from build123d import *

# Parameters (mm, degrees)
F1_DEPTH  = 250
F2_R      = 5
F3_DEPTH  = 25
F5_DEPTH  = 25
F7_DEPTH  = 25
F10_DEPTH = 100


with BuildPart() as f1:
    # F0 (on Front) → F1 (new body)
    with BuildSketch(Plane.XZ):
        Polygon((-47.1529836208, 41.1845914816), (-77.1529836208, 41.1845914816), (-77.1529836208, 38.1845914816), (-47.1529836208, 38.1845914816), (-47.1529836208, 11.1845914816), (27.0837845569, -25.3437928188), (45.465561148, -49.0526580248), (47.8364476686, -50.2144803657), (67.8364476686, -50.2144803657), (67.8364476686, -47.2144803657), (47.8364476686, -47.2144803657), (28.3516393422, -22.6248694577), (-44.1529836208, 11.1845914816), (-44.1529836208, 41.1845914816), align=None)
    extrude(amount=F1_DEPTH)

    # F2 (on face) → F3 (cut)
    with BuildSketch(Plane.XY.offset(41.1845914816)):
        with Locations((-61.1529836208, -30)):
            Circle(F2_R)
        with Locations((-61.1529836208, -125)):
            Circle(F2_R)
        with Locations((-61.1529836208, -220)):
            Circle(F2_R)
    extrude(amount=-F3_DEPTH, mode=Mode.SUBTRACT)

    # F4 (on face) → F5 (cut)
    with BuildSketch(Plane.XY.offset(41.1845914816)):
        with BuildLine():
            ThreePointArc((-77.1529836208, -25), (-69.8306531504, -7.3223304703), (-52.1529836208, 0))
            Line((-52.1529836208, 0), (-77.1529836208, 0))
            Line((-77.1529836208, 0), (-77.1529836208, -25))
        make_face()
        with BuildLine():
            Line((-77.1529836208, -250), (-52.1529836208, -250))
            ThreePointArc((-52.1529836208, -250), (-69.8306531504, -242.6776695297), (-77.1529836208, -225))
            Line((-77.1529836208, -225), (-77.1529836208, -250))
        make_face()
    extrude(amount=-F5_DEPTH, mode=Mode.SUBTRACT)

    # F6 (on face) → F7 (cut)
    with BuildSketch(Plane.XY.offset(41.1845914816)):
        with BuildLine():
            Line((-58.6529836208, -40), (-63.6529836208, -40))
            ThreePointArc((-63.6529836208, -40), (-67.1885175267, -41.4644660941), (-68.6529836208, -45))
            Line((-68.6529836208, -45), (-68.6529836208, -110))
            ThreePointArc((-68.6529836208, -110), (-67.1885175267, -113.5355339059), (-63.6529836208, -115))
            Line((-63.6529836208, -115), (-58.6529836208, -115))
            ThreePointArc((-58.6529836208, -115), (-55.1174497148, -113.5355339059), (-53.6529836208, -110))
            Line((-53.6529836208, -110), (-53.6529836208, -45))
            ThreePointArc((-53.6529836208, -45), (-55.1174497148, -41.4644660941), (-58.6529836208, -40))
        make_face()
        with BuildLine():
            Line((-58.6529836208, -135), (-63.6529836208, -135))
            ThreePointArc((-63.6529836208, -135), (-67.1885175267, -136.4644660941), (-68.6529836208, -140))
            Line((-68.6529836208, -140), (-68.6529836208, -205))
            ThreePointArc((-68.6529836208, -205), (-67.1885175267, -208.5355339059), (-63.6529836208, -210))
            Line((-63.6529836208, -210), (-58.6529836208, -210))
            ThreePointArc((-58.6529836208, -210), (-55.1174497148, -208.5355339059), (-53.6529836208, -205))
            Line((-53.6529836208, -205), (-53.6529836208, -140))
            ThreePointArc((-53.6529836208, -140), (-55.1174497148, -136.4644660941), (-58.6529836208, -135))
        make_face()
    extrude(amount=-F7_DEPTH, mode=Mode.SUBTRACT)

    # F9 (on offset) → F10 (cut)
    with BuildSketch(Plane(origin=(6.9634072107, 0, 14.9330749537), x_dir=(0.906307787, 0, -0.4226182617), z_dir=(0.4226182617, 0, 0.906307787))):
        with BuildLine():
            Line((15, -15), (-15, -15))
            ThreePointArc((-15, -15), (-22.0710678119, -17.9289321881), (-25, -25))
            Line((-25, -25), (-25, -80))
            ThreePointArc((-25, -80), (-22.0710678119, -87.0710678119), (-15, -90))
            Line((-15, -90), (15, -90))
            ThreePointArc((15, -90), (22.0710678119, -87.0710678119), (25, -80))
            Line((25, -80), (25, -25))
            ThreePointArc((25, -25), (22.0710678119, -17.9289321881), (15, -15))
        make_face()
        with BuildLine():
            Line((15, -160), (-15, -160))
            ThreePointArc((-15, -160), (-22.0710678119, -162.9289321881), (-25, -170))
            Line((-25, -170), (-25, -225))
            ThreePointArc((-25, -225), (-22.0710678119, -232.0710678119), (-15, -235))
            Line((-15, -235), (15, -235))
            ThreePointArc((15, -235), (22.0710678119, -232.0710678119), (25, -225))
            Line((25, -225), (25, -170))
            ThreePointArc((25, -170), (22.0710678119, -162.9289321881), (15, -160))
        make_face()
    extrude(amount=-F10_DEPTH, mode=Mode.SUBTRACT)


solid = f1.part
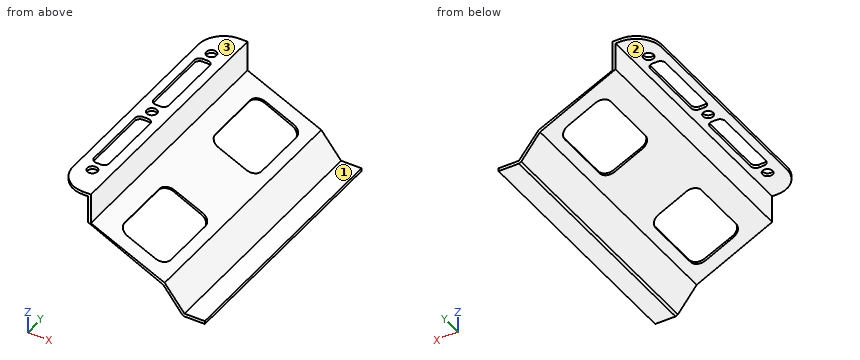
Build history of the part. All positions in model axes, mm. Face numbers are marked on the shaded views. A direction names the side the tool comes from. Round coordinates to 2 decimals unless told otherwise and drop trailing zeros. Loops run counter-clockwise (first coordinate to the right, second up) from the corner with the lowest first, then second, coordinate; pieces in that order, holes last. Notation, with made-up numbers: (42.5, -12.75) -> (63.5, -12.75) arc R20 cw to (63.5, 19.25) -> close; hole circle Ø11 at (54, 74.25). An arc over 180 degrees is marked (long way). One line per item, written item: value. Start each with the question number.
Q1. Cut at A-A on y = -95. List the corners of the cut face in (x, z), plus the area to 3 significant figures.
Q2. Cut at B-B on x = -6. List the corners of the cut face in (y, z).
Q3. Probe line 1 along Z through (x, y) = (54.5, -59.5); line 2 along X through (y, z) = (-179, 36.5); line 3 along X through (y, z) = (-231.5, -24.5). List the from-to ranges inside material, lowest first.
Q4. 3-axis set-ups, long thin cutter, end or side, ignore diameter. For the marked faces 1, 2 and 3: which of +Z, -Z, +X, -X, +Y, -Y reach the whole face in a straight line?
Q5. Cut at C-C on y = -220. List the corners of the cut face in (x, z).
Q6. Drop flat-ended pins along their axis: pin 1 Ø3.5 at (y, z) = (-70.5, 39.5) entering from +X; pin 2 Ø8 at (x, z) = (5.5, -22) entering from -Y; pin 3 Ø8 at (y, z) = (-195, -25.5) entering from -X; pin 4 Ø5 at (x, y) = (-12, -89) entering from -Z. Give the stop position or say it passes through.
Q7. Cut at D-D on z = -10. List the corners of the cut face in (x, y).
Computed:
1. outline: (-77.15, 38.18) -> (-68.65, 38.18) -> (-68.65, 41.18) -> (-77.15, 41.18) -> close; (-53.65, 38.18) -> (-47.15, 38.18) -> (-47.15, 11.18) -> (27.08, -25.34) -> (45.47, -49.05) -> (47.84, -50.21) -> (67.84, -50.21) -> (67.84, -47.21) -> (47.84, -47.21) -> (28.35, -22.62) -> (-44.15, 11.18) -> (-44.15, 41.18) -> (-53.65, 41.18) -> close
1. area: 460 mm²
2. outline: (-250, -9.06) -> (-235, -9.06) -> (-235, -6.61) -> (-250, -6.61) -> close; (-160, -9.06) -> (-90, -9.06) -> (-90, -6.61) -> (-160, -6.61) -> close; (-15, -9.06) -> (0, -9.06) -> (0, -6.61) -> (-15, -6.61) -> close
3. line 1: -50.21 to -47.21
3. line 2: -47.15 to -44.15
3. line 3: 25.37 to 29.84
4. face 1: +Z, +X, +Y, -Y
4. face 2: -Z, -X, +Y, -Y
4. face 3: +Z, +X, -X, +Y, -Y
5. outline: (-77.15, 38.18) -> (-66.15, 38.18) -> (-66.15, 41.18) -> (-77.15, 41.18) -> close; (-56.15, 38.18) -> (-47.15, 38.18) -> (-47.15, 11.18) -> (-26.99, 1.27) -> (-26.26, 2.84) -> (-44.15, 11.18) -> (-44.15, 41.18) -> (-56.15, 41.18) -> close; (17.88, -20.81) -> (27.08, -25.34) -> (45.47, -49.05) -> (47.84, -50.21) -> (67.84, -50.21) -> (67.84, -47.21) -> (47.84, -47.21) -> (28.35, -22.62) -> (19.06, -18.29) -> close
6. pin 1: x = -44.15
6. pin 2: through
6. pin 3: x = 19.27
6. pin 4: z = -7.24
7. outline: (-4.1, -250) -> (1.28, -250) -> (1.28, -235) -> (-4.1, -235) -> close; (-4.1, -160) -> (1.28, -160) -> (1.28, -90) -> (-4.1, -90) -> close; (-4.1, -15) -> (1.28, -15) -> (1.28, 0) -> (-4.1, 0) -> close
